The listing builds one solid part. Answer for the finished solid, in the listing's coordinates (mm). A direction names the side the tool comes from. Give positions to 0.01 mm unless a question says otherwise; leave off trailing zeros. Write each loop counter-clockwise with the first axis right and the second up, starting at its lowest first coordinate (ties: lowest second). Pieces come first, ordered by that corner, then holes. Notation, with made-up numbers: (-2.75, -16) - (18.25, -16) arc R30 cw to (18.25, 16) - close; hole circle Ø11 at (-3, -28.5). An arc over 180 degrees is marked (long way). Use a Markdown table: item, result. Add a question column.
from build123d import *

# Parameters (mm, degrees)
F0_R      = 21.5
F1_DEPTH  = 40
F2_R      = 5
F3_R      = 21.5
F4_DEPTH  = 40
F5_SIZE2  = 7.5
F5_SIZE   = 40
F6_DEPTH  = 10
F7_R      = 10
F10_R     = 4.9
F11_DEPTH = 75
F12_R     = 16.5
F13_DEPTH = 5
F14_R     = 3.1
F15_DEPTH = 85.001
F16_R     = 45.5023146051
F16_R_2   = 12.5
F17_DEPTH = 100
F18_W     = 86.4328397527
F18_H     = 43.3590536159
F19_DEPTH = 25
F20_SIZE  = 1
F21_R     = 4.9
F21_R_2   = 3.1
F22_DEPTH = 2.5


with BuildPart() as f1:
    # F0 (on Top) → F1 (new body)
    with BuildSketch(Plane.XY):
        Circle(F0_R)
    extrude(amount=F1_DEPTH)

    # F2
    f2_edges = [f1.edges().sort_by_distance(p)[0] for p in [
        (-21.5, 0, 40),
    ]]
    fillet(f2_edges, radius=F2_R)

    # F3 (on face) → F4 (join)
    with BuildSketch(Plane(origin=(0, 0, 0), x_dir=(1, 0, 0), z_dir=(0, 0, -1))):
        Circle(F3_R)
    extrude(amount=F4_DEPTH)

    # F5
    f5_edges = [f1.edges().sort_by_distance(p)[0] for p in [
        (-21.5, 0, -40),
    ]]
    chamfer(f5_edges, length=F5_SIZE, length2=F5_SIZE2)

    # F6 (add): a face of the model
    f6_faces = [f1.faces().sort_by_distance(p)[0] for p in [
        (0, 0, -40),
    ]]
    extrude(f6_faces, amount=F6_DEPTH)

    # F7
    f7_edges = [f1.edges().sort_by_distance(p)[0] for p in [
        (-21.5, 0, 0),
    ]]
    fillet(f7_edges, radius=F7_R)

    # F8 (on Right) → F9 (revolve, cut)
    with BuildSketch(Plane.YZ):
        Polygon((-7.5, -40.5), (-17.4298945979, -40.5), (-17.4298945979, -47.5), (-17.4298945979, -53.659953177), (-10, -53.659953177), (-10, -47.5), (-7.5, -47.5), align=None)
    revolve(axis=Axis((0, 0, -53.4000843763), (0, 0, -1)), mode=Mode.SUBTRACT)

    # F10 (on face) → F11 (cut)
    with BuildSketch(Plane(origin=(0, 0, -50), x_dir=(1, 0, 0), z_dir=(0, 0, -1))):
        Circle(F10_R)
    extrude(amount=-F11_DEPTH, mode=Mode.SUBTRACT)

    # F12 (on face) → F13 (cut)
    with BuildSketch(Plane.XY.offset(40)):
        Circle(F12_R)
    extrude(amount=-F13_DEPTH, mode=Mode.SUBTRACT)

    # F14 (on face) → F15 (cut, through all)
    with BuildSketch(Plane.XY.offset(35)):
        Circle(F14_R)
    extrude(amount=-F15_DEPTH, mode=Mode.SUBTRACT)

    # F16 (on face) → F17 (cut)
    with BuildSketch(Plane(origin=(0, 0, -50), x_dir=(1, 0, 0), z_dir=(0, 0, -1))):
        Circle(F16_R)
        Circle(F16_R_2, mode=Mode.SUBTRACT)
    extrude(amount=-F17_DEPTH, mode=Mode.SUBTRACT)

    # F18 (on Front) → F19 (cut, symmetric)
    with BuildSketch(Plane.XZ):
        with Locations((1.7612818629, 46.679526808)):
            Rectangle(F18_W, F18_H)
    extrude(amount=F19_DEPTH, both=True, mode=Mode.SUBTRACT)

    # F20
    f20_edges = [f1.edges().sort_by_distance(p)[0] for p in [
        (-12.5, 0, 25),
    ]]
    chamfer(f20_edges, length=F20_SIZE)

    # F21 (on face) → F22 (join)
    with BuildSketch(Plane.XY.offset(25)):
        Circle(F21_R)
        Circle(F21_R_2, mode=Mode.SUBTRACT)
    extrude(amount=-F22_DEPTH)


solid = f1.part
1. For a pull along X with two mould halves and no side action, classify faces 4 (the flat face through (2, -5, -50)), 5 (the cylindrical face through (-0.33, 7.493, -43.951)), 6 (the cylindrical face through (1.43, -2.75, 23.77)) as released by +X, released by -X, zero draft, split by the parting line, or undercut.
2. The part is cut by section A-A (x = 0). Give the vertices of the cut face in (y, z), and give its area (3 significant figures).
3. The part is cut by section C-C (z = -26). Give the vertices of the cut face in (x, y).
4. Consider L1, parallel to Z at x = -5.5, y = -5.25; L2, parallel to Y at x = 0, z = 23.7; L3, parallel to X at y = 0, z = -23. Determine where each line is inside the solid, lowest interval first. Write a range as [from, to].
5. Which of the six approach directions +Z, -Z, +X, -X, +Y, -Y give full straight-line access (tool end or side, diameter ignored) to faces 1 (the cylindrical face through (11.923, -3.755, -8.701)), 2 (the cylindrical face through (-1.062, 4.783, -14.258)), 3 (the flat face through (8, 0, -40.5))?
6. Given P1, Ø5, axis at x = 0.5, y = -1, coming from the -Z side; P2, Ø6, axis at y = 7, z = -26, coming from the -X side; P3, Ø1.5, axis at x = 5.5, z = -12.5, coming from the +Y side, each flat-ended and moving along its own axis, determine where each tip first touches the part or whether it passes through.
Check values:
| question | item | result |
|---|---|---|
| 1 | face 4 | zero draft |
| 1 | face 5 | split by the parting line |
| 1 | face 6 | undercut |
| 2 | outline | (-12.5, -40.5) - (-7.5, -40.5) - (-7.5, -47.5) - (-10, -47.5) - (-10, -50) - (-4.9, -50) - (-4.9, 22.5) - (-3.1, 22.5) - (-3.1, 25) - (-11.5, 25) - (-12.5, 24) - close; (3.1, 22.5) - (4.9, 22.5) - (4.9, -50) - (10, -50) - (10, -47.5) - (7.5, -47.5) - (7.5, -40.5) - (12.5, -40.5) - (12.5, 24) - (11.5, 25) - (3.1, 25) - close |
| 2 | area | 1,070 mm2 |
| 3 | outline | circle Ø25 at (0, 0); hole circle Ø9.8 at (0, 0) |
| 4 | L1 | z = [-50, -47.5], [-40.5, 25] |
| 4 | L2 | y = [-12.5, -3.1], [3.1, 12.5] |
| 4 | L3 | x = [-12.5, -4.9], [4.9, 12.5] |
| 5 | face 1 | +Z, -Z |
| 5 | face 2 | -Z |
| 5 | face 3 | none |
| 6 | P1 | stops at z = 22.5 |
| 6 | P2 | stops at x = -11.84 |
| 6 | P3 | stops at y = 11.56 |
